The listing builds one solid part. Answer for the finished solid, in the listing's coordinates (mm). A direction names the side the tool comes from. Coordinates: 2 decimals unless noted, no trailing zeros. Order: outer loops, then holes, each group sorted by start corner. A loop starts at its lowest first (then second) coordinate and runs counter-clockwise, first axis right, second up. Notation, with made-up numbers: (61, -16) -> (69, -16) arc R27 cw to (69, 20) -> close; hole circle Ø10 at (74.25, 23). An arc over 180 degrees is marked (long way). Answer in a Markdown table with one row per item. Add a question column.
Autodesk Fusion 360 part; units mm, degrees
sketch "Esboço1" plane through (0, 0, 0) normal (0, 0, 1) x (1, 0, 0)
  arc A0 (21, 37) -> (21, 15) centre (21, 26) ccw
  line L0 (1.9999, 62) -> (2, 62)
  line L1 (2, 7) -> (2, 62)
  line L2 (21, 37) -> (28, 37)
  line L3 (28, 37) -> (28, 42)
  line L4 (28, 42) -> (22, 42)
  line L5 (22, 42) -> (22, 54)
  line L6 (22, 54) -> (28, 54)
  line L7 (28, 54) -> (28, 62)
  line L8 (28, 62) -> (1.9999, 62)
  line L9 (21, 15) -> (28, 15)
  line L10 (28, 15) -> (28, 6.9481)
  line L11 (28, 6.9481) -> (2, 7)
  dimension "d13" = 11
  dimension "d18" = 6
  dimension "d19" = 12
  dimension "d21" = 8
extrude "Extrusão1" add sketch "Esboço1" along normal blind 30
hole "Furo1" at (2, 48, 15) direction (1, 0, 0) diameter 4 depth 40 tip angle 180
hole "Furo2" at (2, 11, 15) direction (1, 0, 0) diameter 4 depth 40 tip angle 180
fillet "Arredondamento1" radius 1.5 8 edges at (2, 34.5, 30) (15, 6.9741, 30) (2, 7, 15) (15, 6.9741, 0) (2, 34.5, 0) (2, 62, 15) (15, 62, 0) (15, 62, 30)
sketch "Esboço2" plane through (2, 0, 0) normal (-1, 0, 0) x (0, -1, 0)
  circle A0 centre (-48, 15) radius 2
  circle A1 centre (-11, 15) radius 2
  line L0 (-60.5, 1.5) -> (-8.497, 1.5)
  line L1 (-8.497, 1.5) -> (-8.497, 28.5)
  line L2 (-8.497, 28.5) -> (-60.5, 28.5)
  line L3 (-60.5, 28.5) -> (-60.5, 1.5)
  circle A2 centre (-48, 15) radius 5
extrude "Extrusão2" cut sketch "Esboço2" against normal blind 15 contours A2
Q1. Straight lines are drawn through the part: line 1 (Y direction, x = 25, z = 5); line 2 (Z direction, x = 20.25, y = 48); line 3 (Y direction, x = 23.75, z = 16.5). For each, find the intervals that lie inside material, in ascending order.
Q2. For faces 1 (the face through (25, 54, 15)), 2 (the face through (17, 45.8, 15.1)), determine the directions among +Z, -Z, +X, -X, +Y, -Y from which every point of the face is accessible in a straight line to the end or side of a thin tool.
Q3. A cutting plane is placed at C-C (z = 15). Determine the outline of the cut face in (x, y), then the cut area to 3 significant figures.
Q4. A cutting plane is placed at A-A (z = 22.5). Determine the outline of the cut face in (x, y), then the cut area to 3 significant figures.
Q5. Given pin 1 (4 mm diameter, centred on x = 8.5, z = 22, fed in from -Y); pin 2 (2 mm diameter, centred on y = 32.5, z = 20, fed in from +X); pin 3 (3.5 mm diameter, centred on y = 46.5, z = 19.5, fed in from +X), each flat-ended and moving along its own axis, determine where each tip first touches the part or whether it passes through.
Q6. A cutting plane is placed at B-B (x = 12.75). State how many separate pieces and enclosed holes the cut face has, then the cut area to 3 significant figures.
Q7. Determine the mould class of faces 3 (the face through (15.182, 9.648, 13.526)), 4 (the face through (15.58, 7.42, 0.43)), 5 (the face through (16, 62, 15)) for opening direction Y: +Y half, -Y half, draft (parallel to the pull), parting line (faces both ways), or undercut.
Returned:
| question | item | result |
|---|---|---|
| 1 | line 1 | y = 6.95 to 15, 37 to 42, 54 to 62 |
| 1 | line 2 | z = 0 to 13, 17 to 30 |
| 1 | line 3 | y = 6.96 to 9.68, 12.32 to 15, 37 to 42, 54 to 62 |
| 2 | face 1 | +Z, -Z, +X |
| 2 | face 2 | -X |
| 3 | outline | (2, 8.5) arc R1.5 ccw to (3.5, 7) -> (28, 6.95) -> (28, 9) -> (2, 9) -> close; (2, 13) -> (28, 13) -> (28, 15) -> (21, 15) arc R11 cw to (21, 37) -> (28, 37) -> (28, 42) -> (22, 42) -> (22, 46) -> (17, 46) -> (17, 43) -> (2, 43) -> close; (2, 53) -> (17, 53) -> (17, 50) -> (22, 50) -> (22, 54) -> (28, 54) -> (28, 62) -> (3.5, 62) arc R1.5 ccw to (2, 60.5) -> close |
| 3 | area | 740 mm² |
| 4 | outline | (2, 8.5) arc R1.5 ccw to (3.5, 7) -> (28, 6.95) -> (28, 15) -> (21, 15) arc R11 cw to (21, 37) -> (28, 37) -> (28, 42) -> (22, 42) -> (22, 54) -> (28, 54) -> (28, 62) -> (3.5, 62) arc R1.5 ccw to (2, 60.5) -> close |
| 4 | area | 1,010 mm² |
| 5 | pin 1 | stops at y = 6.98 |
| 5 | pin 2 | stops at x = 12.95 |
| 5 | pin 3 | stops at x = 22 |
| 6 | separate pieces | 2 |
| 6 | enclosed holes | 2 |
| 6 | area | 1,120 mm² |
| 7 | face 3 | undercut |
| 7 | face 4 | -Y half |
| 7 | face 5 | +Y half |
